from build123d import *

# Parameters (mm, degrees)
SKETCH_1_R      = 1.5
SKETCH_1_R_2    = 0.45
EXTRUDE_1_DEPTH = 1
EXTRUDE_START   = -0.01
SKETCH_1_3_R    = 2
SKETCH_1_3_R_2  = 1.5
SKETCH_1_3_R_3  = 0.95
SKETCH_1_3_R_4  = 0.45
EXTRUDE_2_DEPTH = 1.02
SKETCH_2_W      = 4.5
SKETCH_2_H      = 2.5
EXTRUDE_3_DEPTH = 1
SKETCH_3_W      = 1.6
SKETCH_3_H      = 0.85
SKETCH_3_W_2    = 0.85
SKETCH_3_H_2    = 1.6
EXTRUDE_4_DEPTH = 0.8
SKETCH_3_3_W    = 0.85
SKETCH_3_3_H    = 1.6
SKETCH_3_3_W_2  = 1.8
SKETCH_3_3_H_2  = 3
EXTRUDE_5_DEPTH = 0.5
SKETCH_3_4_W    = 3
SKETCH_3_4_H    = 1.5
SKETCH_3_4_W_2  = 2
SKETCH_3_4_H_2  = 1.2
EXTRUDE_6_DEPTH = 1


with BuildPart() as part:
    # Sketch 1 → Extrude 1 (new body)
    with BuildSketch(Plane(origin=(0, 0, 0), x_dir=(1, 0, 0), z_dir=(0, 1, 0))):
        with BuildLine():
            Line((8, -5.5), (-8, -5.5))
            Line((-8, -5.5), (-8, -2.75))
            Line((-8, -2.75), (-9.75, -2.75))
            ThreePointArc((-9.75, -2.75), (-12.5, 0), (-9.75, 2.75))
            Line((-9.75, 2.75), (-8, 2.75))
            Line((-8, 2.75), (-8, 5.5))
            Line((-8, 5.5), (8, 5.5))
            Line((8, 5.5), (8, 2.75))
            Line((8, 2.75), (9.75, 2.75))
            ThreePointArc((9.75, 2.75), (12.5, 0), (9.75, -2.75))
            Line((9.75, -2.75), (8, -2.75))
            Line((8, -2.75), (8, -5.5))
        make_face()
        with Locations((-9.75, 0)):
            Circle(SKETCH_1_R, mode=Mode.SUBTRACT)
        with Locations((9.75, 0)):
            Circle(SKETCH_1_R, mode=Mode.SUBTRACT)
        with Locations((-6.5, -4)):
            Circle(SKETCH_1_R_2, mode=Mode.SUBTRACT)
        with Locations((-3.96, -4)):
            Circle(SKETCH_1_R_2, mode=Mode.SUBTRACT)
        with Locations((-1.42, -4)):
            Circle(SKETCH_1_R_2, mode=Mode.SUBTRACT)
        with Locations((1.12, -4)):
            Circle(SKETCH_1_R_2, mode=Mode.SUBTRACT)
        with Locations((3.66, -4)):
            Circle(SKETCH_1_R_2, mode=Mode.SUBTRACT)
        with Locations((6.2, -4)):
            Circle(SKETCH_1_R_2, mode=Mode.SUBTRACT)
    extrude(amount=EXTRUDE_1_DEPTH)

    # Sketch 1_3 → Extrude 2 (add)
    with BuildSketch(Plane(origin=(0, 0, 0), x_dir=(1, 0, 0), z_dir=(0, 1, 0)).offset(EXTRUDE_START)):
        with Locations((-9.75, 0)):
            Circle(SKETCH_1_3_R)
        with Locations((-9.75, 0)):
            Circle(SKETCH_1_3_R_2, mode=Mode.SUBTRACT)
        with Locations((-6.5, -4)):
            Circle(SKETCH_1_3_R_3)
        with Locations((-6.5, -4)):
            Circle(SKETCH_1_3_R_4, mode=Mode.SUBTRACT)
        with Locations((-3.96, -4)):
            Circle(SKETCH_1_3_R_3)
        with Locations((-3.96, -4)):
            Circle(SKETCH_1_3_R_4, mode=Mode.SUBTRACT)
        with Locations((-1.42, -4)):
            Circle(SKETCH_1_3_R_3)
        with Locations((-1.42, -4)):
            Circle(SKETCH_1_3_R_4, mode=Mode.SUBTRACT)
        with Locations((1.12, -4)):
            Circle(SKETCH_1_3_R_3)
        with Locations((1.12, -4)):
            Circle(SKETCH_1_3_R_4, mode=Mode.SUBTRACT)
        with Locations((3.66, -4)):
            Circle(SKETCH_1_3_R_3)
        with Locations((3.66, -4)):
            Circle(SKETCH_1_3_R_4, mode=Mode.SUBTRACT)
        with Locations((6.2, -4)):
            Circle(SKETCH_1_3_R_3)
        with Locations((6.2, -4)):
            Circle(SKETCH_1_3_R_4, mode=Mode.SUBTRACT)
        with Locations((9.75, 0)):
            Circle(SKETCH_1_3_R)
        with Locations((9.75, 0)):
            Circle(SKETCH_1_3_R_2, mode=Mode.SUBTRACT)
    extrude(amount=EXTRUDE_2_DEPTH)

    # Sketch 2 → Extrude 3 (add)
    with BuildSketch(Plane(origin=(0, 1, 0), x_dir=(1, 0, 0), z_dir=(0, 1, 0))):
        with Locations((0, 2)):
            Rectangle(SKETCH_2_W, SKETCH_2_H)
    extrude(amount=EXTRUDE_3_DEPTH)

    # Sketch 3 → Extrude 4 (add)
    with BuildSketch(Plane.XZ):
        with Locations((-5.2, 1.875)):
            Rectangle(SKETCH_3_W, SKETCH_3_H)
        with Locations((-1.69, -3.7)):
            Rectangle(SKETCH_3_W_2, SKETCH_3_H_2)
        with Locations((0, -3.7)):
            Rectangle(SKETCH_3_W_2, SKETCH_3_H_2)
        with Locations((1.69, -3.7)):
            Rectangle(SKETCH_3_W_2, SKETCH_3_H_2)
    extrude(amount=EXTRUDE_4_DEPTH)

    # Sketch 3_3 → Extrude 5 (add)
    with BuildSketch(Plane.XZ):
        with Locations((6.575, -0.7)):
            Rectangle(SKETCH_3_3_W, SKETCH_3_3_H)
        with Locations((5.075, -0.7)):
            Rectangle(SKETCH_3_3_W, SKETCH_3_3_H)
        with Locations((-2.1, 1)):
            Rectangle(SKETCH_3_3_W_2, SKETCH_3_3_H_2)
    extrude(amount=EXTRUDE_5_DEPTH)

    # Sketch 3_4 → Extrude 6 (add)
    with BuildSketch(Plane.XZ):
        with Locations((-5.5, -1.25)):
            Rectangle(SKETCH_3_4_W, SKETCH_3_4_H)
        with Locations((1.5, 0.9)):
            Rectangle(SKETCH_3_4_W_2, SKETCH_3_4_H_2)
    extrude(amount=EXTRUDE_6_DEPTH)


solid = part.part
Source: CAD feature listing. Evaluate the final solid. Frame: model axes, mm. A direction names the side the tool comes from. Coordinates: 2 decimals unless noted, no trailing zeros. Use a Markdown table: item, result.
1) First-contact query: pin 1 Ø0.6 at (x, z) = (6, 3.5) entering from +Y; pin 2 Ø0.8 at (y, z) = (0.5, -3.5) entering from +X; pin 3 Ø0.5 at (x, y) = (0, 1.5) entering from -Z. Flat tips, straight axial feed; report the tip coordinate or a pass-through.
Conclusion:
| item | result |
|---|---|
| pin 1 | stops at y = 1.01 |
| pin 2 | stops at x = 8 |
| pin 3 | stops at z = -3.25 |
2) Ray query, L1, parallel to X at y = 0.25, z = 0; L2, parallel to Z at x = 6.2, y = 0.8; L3, parallel to X at y = -0.7, z = -1. Return the intervals inside material, ascending.
Conclusion:
| item | result |
|---|---|
| L1 | x = -12.5 to -11.25, -8.25 to 8.25, 11.25 to 12.5 |
| L2 | z = -5.5 to 3.55, 4.45 to 5.5 |
| L3 | x = -7 to -4 |
3) Section B-B, the plane y = 0.4. Give the number of separate pieces and of enclosed holes in the cut face, then the cut area to 3 significant figures.
Conclusion:
| item | result |
|---|---|
| separate pieces | 1 |
| enclosed holes | 8 |
| area | 201 mm^2 |
4) Reachability of faces 1 (the flat face through (-2, -0.5, 1)), 2 (the flat face through (3, 1.01, 4)), 3 (the flat face through (7, -0.01, 4)), 4 (the flat face through (0.1, 0.5, 5.5)), 5 (the flat face through (8, 0.5, -4.1)) from +Z, -Z, +X, -X, +Y, -Y: full face, straight path, thin tool, end or side. Return the list, or none.
Conclusion:
| item | result |
|---|---|
| face 1 | +Z, -Y |
| face 2 | +Z, -Z, +X, -X, +Y |
| face 3 | +Z, +X, -X, -Y |
| face 4 | +Z, +X, -X, +Y, -Y |
| face 5 | -Z, +X, +Y, -Y |
5) Mould query, pull axis Z, two halves, no side actions, for faces 6 (the cylindrical face through (-12.5, 0.5, 0.1)), 7 (the flat face through (1.7, -0.8, -3.7)), 8 (the cylindrical face through (-1.18, 0.49, 3.62)). Classes: pulls with the +Z half, pulls with the -Z half, needs draft (parallel to the pull), parting line crosses it, or undercut.
Conclusion:
| item | result |
|---|---|
| face 6 | parting line crosses it |
| face 7 | needs draft |
| face 8 | undercut |
